Part print with two shaded views. Sizes in mm from the minimum x, y, z corner. A direction names the side the tool comes from. Round coordinates to 2 decimals unless told otherwise and drop trailing zeros. Loops run counter-clockwise (first coordinate to the right, second up) from the corner with the lowest first, then second, coordinate; pieces in that order, holes last. Notation, with made-up numbers: (48.5, 54) - (102.5, 54) arc R9 cw to (102.5, 65) - close; hole circle Ø11 at (-6.75, 40). An arc over 180 degrees is marked (long way). Use a Markdown table: item, result.
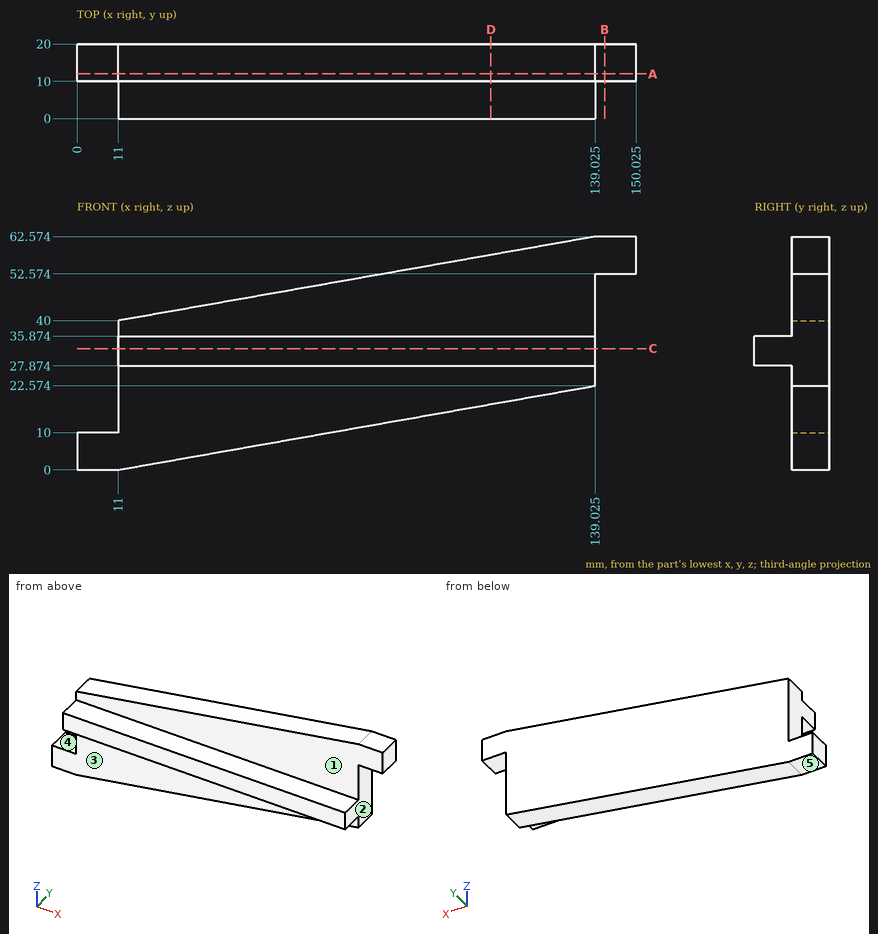
Q1. Probe line 1 (Z direction, x = 69, y = 4); line 2 (Y direction, x = 19, z = 24); line 3 (X direction, y = 4, z = 35.5) (1 decimal). List the from-to ranges inside material, lowest first.
Results found:
| item | result |
|---|---|
| line 1 | z = 27.87 to 35.87 |
| line 2 | y = 10 to 20 |
| line 3 | x = 11 to 139 |
Q2. Cut at C-C, the plane z = 32.5. List the corners of the cut face in (x, y) (1 decimal).
Results found:
| item | result |
|---|---|
| outline | (11, 0) - (139, 0) - (139, 20) - (11, 20) - close |
Q3. Drop flat-ended pins along their axis: pin 1 (2 mm diameter, centred on x = 99, z = 56, fed in from -Y); pin 2 (5 mm diameter, centred on x = 44, y = 3, fed in from +Z); pin 3 (10 mm diameter, centred on y = 9, z = 28.5, fed in from -X); pin 4 (5 mm diameter, centred on x = 22.5, z = 26, fed in from -Y). Give the stop position or say it passes through.
Results found:
| item | result |
|---|---|
| pin 1 | stops at y = 10 |
| pin 2 | stops at z = 35.87 |
| pin 3 | stops at x = 11 |
| pin 4 | stops at y = 0 |
Q4. Cut at D-D, the plane x = 111. List the corners of the cut face in (y, z).
Results found:
| item | result |
|---|---|
| outline | (0, 27.87) - (10, 27.87) - (10, 17.63) - (20, 17.63) - (20, 57.63) - (10, 57.63) - (10, 35.87) - (0, 35.87) - close |
Q5. Cut at A-A, the plane y = 12. List the corners of the cut face in (x, z) (1 decimal), plus the area to 3 significant figures.
Results found:
| item | result |
|---|---|
| outline | (0, 0) - (11, 0) - (139, 22.6) - (139, 52.6) - (150, 52.6) - (150, 62.6) - (139, 62.6) - (11, 40) - (11, 10) - (0, 10) - close |
| area | 5,340 mm2 |
Q6. Cut at B-B, the plane x = 141.5. List the corners of the cut face in (y, z).
Results found:
| item | result |
|---|---|
| outline | (10, 52.57) - (20, 52.57) - (20, 62.57) - (10, 62.57) - close |
Q7. Which spindle directions (+Z, -Z, +X, -X, +Y, -Y) get a long thin tool onto all of the face, cutting with end or side? Do the marked faces 1, 2, 3, 4 and 5. Say none if no direction does.
Results found:
| item | result |
|---|---|
| face 1 | +Z, +X, -X, -Y |
| face 2 | -Z, +X, +Y, -Y |
| face 3 | -Z, +X, -X, -Y |
| face 4 | +Z, -X, +Y, -Y |
| face 5 | -Z, +X, -X, +Y, -Y |
